Read the model definition and answer for the solid it produces. Units are mm, in the model's axes. Face numbers are marked on the shaded views. A direction names the side the tool comes from. Give positions to 0.01 mm unless a question says otherwise; leave off trailing zeros. Order: outer loops, then holes, each group sorted by start corner. A loop starts at its lowest first (then second) coordinate and runs counter-clockwise, first axis right, second up. Notation, with made-up numbers: M -13,33 L 2,33 A20 ccw 2,64 Z; hole C 21.5,75 d8. An arc over 180 degrees is marked long. Write item = value, one per line. Start each with the question number.
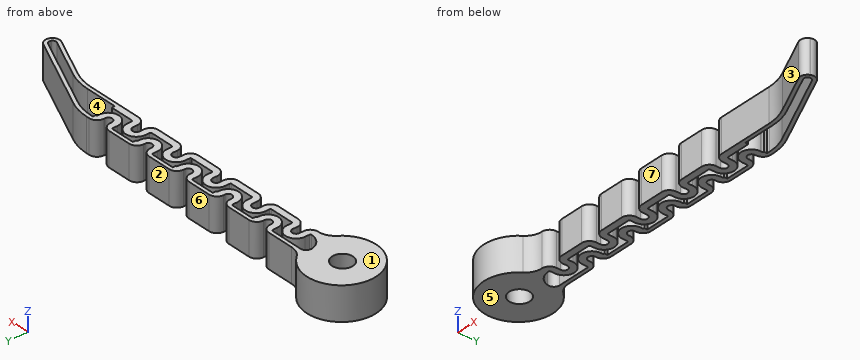
from build123d import *

# Parameters (mm, degrees)
BOSS_EXTRU_1_DEPTH         = 5
CONG_4_R                   = 5
CONG_3_R                   = 15
ENL_V_MAT_EXTRU_5_DEPTH    = 116.769346319
R_P_TITION_LIN_AIRE1_COUNT = 5
R_P_TITION_LIN_AIRE1_PITCH = 14
ENL_V_MAT_EXTRU_6_DEPTH    = 116.769346319
CONG_6_R                   = 2.1


with BuildPart() as part:
    # Esquisse1 → Boss.-Extru.1 (new, symmetric)
    with BuildSketch(Plane.XY):
        with BuildLine():
            Line((9.090688918, 5), (86.842811698, 5))
            Line((86.842811698, 5), (114.721401665, -8))
            Line((114.721401665, -8), (112.90414314, -11.897123484))
            Line((112.90414314, -11.897123484), (95.539805791, -3.8))
            Line((95.539805791, -3.8), (9.654047079, -3.8))
            ThreePointArc((9.654047079, -3.8), (-10.353805189, -0.662829619), (9.090688918, 5))
        make_face()
    extrude(amount=BOSS_EXTRU_1_DEPTH, both=True)

    # Cong_4
    cong_4_edges = [part.edges().sort_by_distance(p)[0] for p in [
        (9.654047079, -3.8, 0),
        (9.090688918, 5, 0),
    ]]
    fillet(cong_4_edges, radius=CONG_4_R)

    # Cong_3
    cong_3_edges = [part.edges().sort_by_distance(p)[0] for p in [
        (95.539805791, -3.8, 0),
        (86.842811698, 5, 0),
    ]]
    fillet(cong_3_edges, radius=CONG_3_R)

    # Esquisse10 → Enl_vement de mati_re-R_volution1 (revolve, cut)
    with BuildSketch(Plane(origin=(0, 0, 0), x_dir=(1, 0, 0), z_dir=(0, 1, 0)), mode=Mode.PRIVATE) as enl_vement_de_mati_re_r_volution1_sk:
        Polygon((0.697564737, 9.975640503), (-0.697564737, -9.975640503), (2.394883818, -10.191885571), (3.790013293, 9.759395434), align=None)
    revolve(enl_vement_de_mati_re_r_volution1_sk.sketch.rotate(Axis((0.697564737, 0, -9.975640503), (0.06975647374413119, 0, -0.9975640502598239)), 180), axis=Axis((0.697564737, 0, -9.975640503), (0.06975647374413119, 0, -0.9975640502598239)), mode=Mode.SUBTRACT)

    # Esquisse8 → Enl_v. mat.-Extru.5 (cut, symmetric)
    with BuildSketch(Plane(origin=(0, 0, -5), x_dir=(-1, 0, 0), z_dir=(0, 0, -1))):
        with BuildLine():
            Line((-17.257562182, -0.15), (-17.257562182, -1.450000033))
            ThreePointArc((-17.257562182, -1.450000033), (-17.945861236, -3.111700945), (-19.607562149, -3.8))
            Line((-19.607562149, -3.8), (-12.607562215, -3.8))
            ThreePointArc((-12.607562215, -3.8), (-14.269263127, -3.111700945), (-14.957562182, -1.450000033))
            Line((-14.957562182, -1.450000033), (-14.957562182, -0.15))
            ThreePointArc((-14.957562182, -0.15), (-16.107562182, 1), (-17.257562182, -0.15))
        make_face()
        with BuildLine():
            Line((-19.607562281, 3.9), (-12.607562215, 3.9))
            Line((-12.607562215, 3.9), (-12.607562215, -1.8))
            ThreePointArc((-12.607562215, -1.8), (-12.855049565, -1.697487383), (-12.957562182, -1.450000033))
            Line((-12.957562182, -1.450000033), (-12.957562182, -0.15))
            ThreePointArc((-12.957562182, -0.15), (-16.107562182, 3), (-19.257562182, -0.15))
            Line((-19.257562182, -0.15), (-19.257562182, -1.450000033))
            ThreePointArc((-19.257562182, -1.450000033), (-19.360074845, -1.69748743), (-19.607562281, -1.8))
            Line((-19.607562281, -1.8), (-26.607562215, -1.8))
            Line((-26.607562215, -1.8), (-26.607562215, 3))
            ThreePointArc((-26.607562215, 3), (-26.360074865, 2.897487383), (-26.257562248, 2.650000033))
            Line((-26.257562248, 2.650000033), (-26.257562248, 2.25))
            ThreePointArc((-26.257562248, 2.25), (-23.107562248, -0.9), (-19.957562248, 2.25))
            Line((-19.957562248, 2.25), (-19.957562248, 3.550000033))
            ThreePointArc((-19.957562248, 3.550000033), (-19.855049631, 3.797487383), (-19.607562281, 3.9))
        make_face()
        with BuildLine():
            Line((-26.607562215, 5), (-19.607562281, 5))
            ThreePointArc((-19.607562281, 5), (-21.269263193, 4.311700945), (-21.957562248, 2.650000033))
            Line((-21.957562248, 2.650000033), (-21.957562248, 2.25))
            ThreePointArc((-21.957562248, 2.25), (-23.107562248, 1.1), (-24.257562248, 2.25))
            Line((-24.257562248, 2.25), (-24.257562248, 2.650000033))
            ThreePointArc((-24.257562248, 2.650000033), (-24.945861302, 4.311700945), (-26.607562215, 5))
        make_face()
    enl_v_mat_extru_5 = extrude(amount=ENL_V_MAT_EXTRU_5_DEPTH, both=True, mode=Mode.SUBTRACT)

    # R_p_tition lin_aire1: Enl_v. mat.-Extru.5 ×5
    with Locations(*[(i * R_P_TITION_LIN_AIRE1_PITCH, 0, 0) for i in range(1, R_P_TITION_LIN_AIRE1_COUNT)]):
        add(enl_v_mat_extru_5, mode=Mode.SUBTRACT)

    # Esquisse9 → Enl_v. mat.-Extru.6 (cut, through all)
    with BuildSketch(Plane(origin=(0, 0, -5), x_dir=(-1, 0, 0), z_dir=(0, 0, -1))):
        with BuildLine():
            Line((-12.607562215, 3.9), (-12.607562215, -1.8))
            ThreePointArc((-12.607562215, -1.8), (-9.766736082, -0.796647883), (-8.186194586, 1.768288211))
            ThreePointArc((-8.186194586, 1.768288211), (-8.5369321, 3.245312267), (-9.906603899, 3.9))
            Line((-9.906603899, 3.9), (-12.607562215, 3.9))
        make_face()
        with BuildLine():
            Line((-83.517391759, 3.9), (-82.607562215, 3.9))
            Line((-82.607562215, 3.9), (-82.607562215, -2.7))
            Line((-82.607562215, -2.7), (-92.214385852, -2.7))
            ThreePointArc((-92.214385852, -2.7), (-95.699063636, -3.081634285), (-99.018539866, -4.208444629))
            Line((-99.018539866, -4.208444629), (-111.465776875, -10.012686569))
            ThreePointArc((-111.465776875, -10.012686569), (-112.23041528, -10.046071403), (-112.794702924, -9.528997044))
            Line((-112.794702924, -9.528997044), (-112.83696475, -9.438366265))
            ThreePointArc((-112.83696475, -9.438366265), (-112.870349583, -8.67372786), (-112.353275224, -8.109440216))
            Line((-112.353275224, -8.109440216), (-89.391785597, 2.59767824))
            ThreePointArc((-89.391785597, 2.59767824), (-86.525902393, 3.570514499), (-83.517391759, 3.9))
        make_face()
    extrude(amount=-ENL_V_MAT_EXTRU_6_DEPTH, mode=Mode.SUBTRACT)

    # Cong_6
    cong_6_edges = [part.edges().sort_by_distance(p)[0] for p in [
        (114.721401665, -8, 0),
        (112.90414314, -11.897123484, 0),
    ]]
    fillet(cong_6_edges, radius=CONG_6_R)


solid = part.part
1) Find section A-A on x = 105. Determine the outline of the cut face in (y, z).
2) Find section B-B on z = -1. Count the separate pieces of the cut face and the enclosed holes in it, plus the area to 3 significant figures.
3) For a pull along Y with two mould halves and no side action, classify the marked faces 4, 5, 6 and 7 as pulls with the +Y half, pulls with the -Y half, needs draft (parallel to the pull), parting line crosses it, or undercut.
4) Each of these flat-tipped pins is pushed along its axis until it touches: P1, Ø5, axis at y = 6.5, z = 2.5, coming from the -X side; P2, Ø2, axis at x = 28.5, z = -0.5, coming from the -Y side; P3, Ø1.4, axis at y = 3, z = 1.5, coming from the -X side. Where does it stop, or does it pass through?
5) Find the intervals of material crossed by probe 1 along X at (y, z) = (-8.75, 0.5); probe 2 along Y at (x, z) = (30, 2.25); probe 3 along X at (y, z) = (-5.25, -1), in increasing order. Write a range as [from, to].
6) For the marked faces 1, 2 and 3, determine the directions among +Z, -Z, +X, -X, +Y, -Y from which every point of the face is accessible in a straight line to the end or side of a thin tool.
Numbers:
q1.outline = M -8.21,-5 L -7,-5 L -7,5 L -8.21,5 Z; M -4.68,-5 L -3.47,-5 L -3.47,5 L -4.68,5 Z
q2.separate_pieces = 1
q2.enclosed_holes = 2
q2.area = 747 mm2
q3.face_4 = undercut
q3.face_5 = needs draft
q3.face_6 = pulls with the +Y half
q3.face_7 = pulls with the -Y half
q4.P1 = -9.57
q4.P2 = -3.62
q4.P3 = -10.12
q5.probe_1 = [-5.57, 5.57], [106.16, 108.76], [112.89, 114.01]
q5.probe_2 = [0.99, 3], [3.9, 5]
q5.probe_3 = [-8.95, 9.09], [98.65, 101.25], [106.22, 108.82]
q6.face_1 = +Z, +X, -X, +Y, -Y
q6.face_2 = +Z, -Z, +X, +Y
q6.face_3 = +Z, -Z, -Y
